Here's how the part is built. I have some questions about the finished solid (model axes, mm). A direction names the side the tool comes from. Coordinates: 2 decimals unless noted, no trailing zeros. Order: outer loops, then holes, each group sorted by start corner. A loop starts at its lowest first (then second) coordinate and runs counter-clockwise, first axis right, second up.
Autodesk Fusion 360 part; units mm, degrees
sketch "Sketch1" plane through (0, 0, 0) normal (0, 0, 1) x (1, 0, 0)
  line L0 (0, 0) -> (0, 45)
  line L1 (0, 45) -> (10, 45)
  line L2 (10, 45) -> (10, 10)
  line L3 (10, 10) -> (100, 10)
  line L4 (100, 10) -> (100, 0)
  line L5 (100, 0) -> (0, 0)
  dimension "d1" = 10
  dimension "d2" = 100
  dimension "d3" = 45
extrude "Extrude1" add sketch "Sketch1" along normal mid plane 100
fillet "Fillet1" radius 20 4 edges at (5, 45, 50) (5, 45, -50) (100, 5, -50) (100, 5, 50)
sketch "Sketch2" plane through (10, 0, 0) normal (1, 0, 0) x (0, 0, -1)
  arc A0 (50, 25) -> (30, 45) centre (30, 25) ccw
  line L0 (30, 45) -> (-30, 45)
  arc A1 (-30, 45) -> (-50, 25) centre (-30, 25) ccw
  line L1 (-50, 25) -> (-50, 10)
  line L2 (-50, 10) -> (50, 10)
  line L3 (50, 10) -> (50, 25)
  circle A2 centre (-30, 25) radius 10
  circle A3 centre (30, 25) radius 10
  dimension "d7" = 20
extrude "Extrude2" cut sketch "Sketch2" against normal through all contours A2 | A3
sketch "Sketch3" plane through (0, 10, 0) normal (0, 1, 0) x (-1, 0, 0)
  arc A0 (-80, 50) -> (-100, 30) centre (-80, 30) ccw
  line L0 (-100, 30) -> (-100, -30)
  arc A1 (-100, -30) -> (-80, -50) centre (-80, -30) ccw
  line L1 (-80, -50) -> (-10, -50)
  line L2 (-10, -50) -> (-10, 50)
  line L3 (-10, 50) -> (-80, 50)
  circle A2 centre (-80, -30) radius 10
  circle A3 centre (-80, 30) radius 10
  dimension "d9" = 20
extrude "Extrude3" cut sketch "Sketch3" against normal through all contours A2 | A3
Q1. We'd pull the mould along X, two halves only. Please class faces 3 (the flat face through (0, 22, -1)), 4 (the cylindrical face through (5.07, 39.297, 43.986)), 5 (the cylindrical face through (90, 5, -30)), 6 (the cylindrical face through (88, 5, 24)): pulls with the +X half, pulls with the -X half, needs draft (parallel to the pull), parting line crosses it, or undercut.
Q2. I need wall thicknesses on L1, parallel to Z at x = 80, y = 4; L2, parallel to Y at x = 3.5, z = -30; L3, parallel to Y at x = 56, z = -30. Which ranges of each line are inside material? Lowest first, please.
Q3. Will these pins go through, and if not, where does the flat tip stop? pin 1 (6 mm diameter, centred on x = 81, z = -38.5, fed in from +Y); pin 2 (10.5 mm diameter, centred on y = 28.5, z = 22, fed in from +X).
Q4. If we section it at A-A on y = 17: Write out the boundary of the cut face in (x, z), then the cut area to 3 significant figures.
Q5. If we section it at D-D on z = 14: Write out the boundary of the cut face in (x, y).
Q6. For faces 1 (the cylindrical face through (5.07, 28, -39.54)), 2 (the flat face through (10, 28, -1)), which set-ups out of +Z, -Z, +X, -X, +Y, -Y let a thin tool reach every point of the face, with its end or its side?
Q7. If we section it at C-C on x = 87: Write out the boundary of the cut face in (y, z) (3 decimals).
Q8. If we section it at B-B on z = -22: Write out the boundary of the cut face in (x, y).
Reply:
1. face 3: pulls with the -X half
1. face 4: needs draft
1. face 5: undercut
1. face 6: undercut
2. L1: z = -50 to -40, -20 to 20, 40 to 50
2. L2: y = 0 to 15, 35 to 45
2. L3: y = 0 to 10
3. pin 1: stops at y = 10
3. pin 2: stops at x = 10
4. outline: (0, -50) - (10, -50) - (10, -36) - (0, -36) - close; (0, -24) - (10, -24) - (10, 24) - (0, 24) - close; (0, 36) - (10, 36) - (10, 50) - (0, 50) - close
4. area: 760 mm2
5. outline: (0, 0) - (100, 0) - (100, 10) - (10, 10) - (10, 45) - (0, 45) - close
6. face 1: +X, -X
6. face 2: +Z, -Z, +X, +Y
7. outline: (0, -48.735) - (10, -48.735) - (10, -37.141) - (0, -37.141) - close; (0, -22.859) - (10, -22.859) - (10, 22.859) - (0, 22.859) - close; (0, 37.141) - (10, 37.141) - (10, 48.735) - (0, 48.735) - close
8. outline: (0, 0) - (74, 0) - (74, 10) - (10, 10) - (10, 19) - (0, 19) - close; (0, 31) - (10, 31) - (10, 45) - (0, 45) - close; (86, 0) - (100, 0) - (100, 10) - (86, 10) - close
